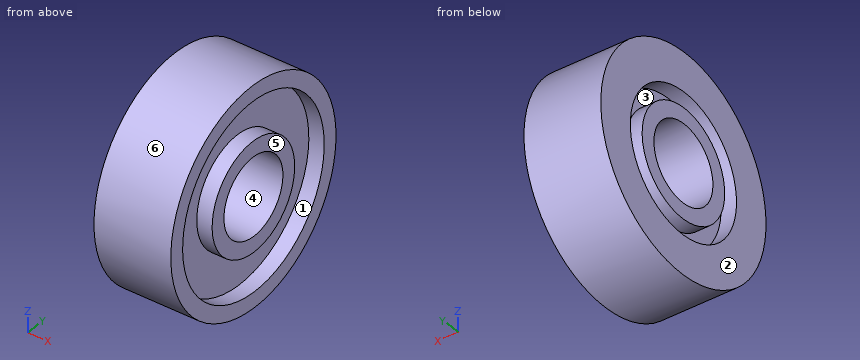
from build123d import *

# Parameters (mm, degrees)
SKETCH_1_R          = 7
SKETCH_1_R_2        = 2.5
EXTRUDE_1_DEPTH     = 2.5
SKETCH_2_R          = 6
SKETCH_2_R_2        = 3.5
CUT_EXTRUDE_1_DEPTH = 1
CUT_EXTRUDE_START   = -1
SKETCH_3_R          = 4.5
SKETCH_3_R_2        = 3.5
CUT_EXTRUDE_2_DEPTH = 1


with BuildPart() as part:
    # 草图1 → 凸台-拉伸1 (new, symmetric)
    with BuildSketch(Plane.YZ):
        with Locations(Location((0, 0, 0), (0, 0, 270))):
            Circle(SKETCH_1_R)
        with Locations(Location((0, 0, 0), (0, 0, 270))):
            Circle(SKETCH_1_R_2, mode=Mode.SUBTRACT)
    extrude(amount=EXTRUDE_1_DEPTH, both=True)

    # 草图2 → 切除-拉伸1 (cut)
    with BuildSketch(Plane(origin=(2.5, 0, 0), x_dir=(0, 0, -1), z_dir=(1, 0, 0))):
        Circle(SKETCH_2_R)
        Circle(SKETCH_2_R_2, mode=Mode.SUBTRACT)
    extrude(amount=-CUT_EXTRUDE_1_DEPTH, mode=Mode.SUBTRACT)

    # 草图3 → 切除-拉伸2 (cut)
    with BuildSketch(Plane.ZY.offset(2.5).offset(CUT_EXTRUDE_START)):
        Circle(SKETCH_3_R)
        with Locations(Location((0, 0, 0), (0, 0, 180))):
            Circle(SKETCH_3_R_2, mode=Mode.SUBTRACT)
    extrude(amount=CUT_EXTRUDE_2_DEPTH, mode=Mode.SUBTRACT)


solid = part.part
Source: CAD feature listing. Evaluate the final solid. Frame: model axes, mm. Face numbers are marked on the shaded views. A direction names the side the tool comes from. Give positions to 0.01 mm unless a question says otherwise; leave off trailing zeros. Write each loop counter-clockwise with the first axis right and the second up, starting at its lowest first coordinate (ties: lowest second). Pieces come first, ordered by that corner, then holes. Notation, with made-up numbers: (50, 21) - (102, 21) arc R13 cw to (102, 43) - close; hole circle Ø8 at (-10.75, 60.25). An arc over 180 degrees is marked (long way). Write item = value, one per line. Start each with the question number.
Q1. Pin query (flat end, axial travel): pin 1 Ø1.5 at (x, z) = (-1.5, -1.5) entering from +Y; pin 2 Ø4 at (y, z) = (0, 0) entering from -X; pin 3 Ø1.5 at (x, z) = (0.5, -5.5) entering from -Y. Return the tip coordinate at first contact, or that it passes through.
Q2. Material intervals for probe 1 along Y at (x, z) = (2, 0); probe 2 along Y at (x, z) = (1.15, 0); probe 3 along Y at (x, z) = (-2.1, 0), sorted ascending.
Q3. Reachability of the marked faces 1, 2 and 3 from +Z, -Z, +X, -X, +Y, -Y: full face, straight path, thin tool, end or side. Return the list, or none.
Q4. Draft query along Z for the marked faces 4, 5 and 6. Return one class per face: +Z half, -Z half, draft (parallel to the pull), parting line (faces both ways), or undercut.
Q5. Cut plane D-D, the plane x = 0. Return loops of the section in (y, z).
Q6. Cut plane C-C, the plane y = -4. Return loops of the section in (x, z).
Q7. Cut plane A-A, the plane z = 0. Return loops of the section in (x, y).
Computed values:
q1.pin_1 = 6.96
q1.pin_2 = through
q1.pin_3 = -5.14
q2.probe_1 = -7 to -6, -3.5 to -2.5, 2.5 to 3.5, 6 to 7
q2.probe_2 = -7 to -2.5, 2.5 to 7
q2.probe_3 = -7 to -4.5, -3.5 to -2.5, 2.5 to 3.5, 4.5 to 7
q3.face_1 = +X
q3.face_2 = +Z, -Z, -X, +Y, -Y
q3.face_3 = -X
q4.face_4 = undercut
q4.face_5 = draft
q4.face_6 = parting line
q5.outline = circle Ø14 at (0, 0); hole circle Ø5 at (0, 0)
q6.outline = (-2.5, -5.74) - (2.5, -5.74) - (2.5, -4.47) - (1.5, -4.47) - (1.5, 4.47) - (2.5, 4.47) - (2.5, 5.74) - (-2.5, 5.74) - (-2.5, 2.06) - (-1.5, 2.06) - (-1.5, -2.06) - (-2.5, -2.06) - close
q7.outline = (-2.5, -7) - (2.5, -7) - (2.5, -6) - (1.5, -6) - (1.5, -3.5) - (2.5, -3.5) - (2.5, -2.5) - (-2.5, -2.5) - (-2.5, -3.5) - (-1.5, -3.5) - (-1.5, -4.5) - (-2.5, -4.5) - close; (-2.5, 2.5) - (2.5, 2.5) - (2.5, 3.5) - (1.5, 3.5) - (1.5, 6) - (2.5, 6) - (2.5, 7) - (-2.5, 7) - (-2.5, 4.5) - (-1.5, 4.5) - (-1.5, 3.5) - (-2.5, 3.5) - close
